Design review of the part built by this model. Coordinates are the model's own, in mm. A direction names the side the tool comes from. Round coordinates to 2 decimals unless told otherwise and drop trailing zeros. Loops run counter-clockwise (first coordinate to the right, second up) from the corner with the lowest first, then second, coordinate; pieces in that order, holes last. Notation, with made-up numbers: (81.25, 50.5) - (87.25, 50.5) arc R38 cw to (87.25, 88.5) - close; hole circle Ø5 at (70.5, -8.75). An arc over 180 degrees is marked (long way). Return JSON: item names as keys, results as strings. Group by question number.
(1) Wall thickness on L1, parallel to Y at x = -1.75, z = 18; L2, parallel to Z at x = 4.25, y = 3.25; L3, parallel to Y at x = 0.75, z = 11: over which ranges is each line inside the solid? List them lowest first. Write a range as [from, to].
(2) Clearance check with flat-ended pins moving along their axes: pin 1 (1.5 mm diameter, centred on y = -5, z = 26.5, fed in from -X); pin 2 (8 mm diameter, centred on y = 2.5, z = 21.5, fed in from +X). State where each tip first meets the part, or that it passes through.
(3) For faces 1 (the flat face through (-3.3, -5.6, 2.7)), 2 (the cylindrical face through (-0.867, -3.905, 22.558)), list the 3-axis set-ups (+Z, -Z, +X, -X, +Y, -Y) from which the entire face can be reached by the end or side of a thin tool; tool diameter is ignored.
(4) We need section A-A, the plane z = 34.5. Write out the cut boundary in (x, y), and give its area (3 significant figures).
from build123d import *

# Parameters (mm, degrees)
F1_DEPTH = 5.5
F2_R     = 4
F3_DEPTH = 35
F4_SIZE  = 0.4


with BuildPart() as f1:
    # F0 (on Top) → F1 (new body)
    with BuildSketch(Plane.XY):
        Polygon((6.5, 3.752777), (0, 7.505553), (-6.5, 3.752777), (-6.5, -3.752777), (0, -7.505553), (6.5, -3.752777), align=None)
    extrude(amount=F1_DEPTH)

    # F2 (on face) → F3 (join)
    with BuildSketch(Plane.XY.offset(5.5)):
        Circle(F2_R)
    extrude(amount=F3_DEPTH)

    # F4
    f4_edges = [f1.edges().sort_by_distance(p)[0] for p in [
        (-4, 0, 40.5),
    ]]
    chamfer(f4_edges, length=F4_SIZE)

    # F5 (on Front) → F6 (revolve, cut)
    with BuildSketch(Plane.XZ):
        Polygon((-11.5, 1), (-11.5, 0), (-6.5, 0), align=None)
    revolve(axis=Axis((0, 0, 5.5), (0, 0, -1)), mode=Mode.SUBTRACT)


solid = f1.part
Solutions:
{
 "1": {"L1": "[-3.6, 3.6]", "L2": "[0, 5.5]", "L3": "[-3.93, 3.93]"},
 "2": {"pin 1": "through", "pin 2": "x = 4"},
 "3": {"face 1": "+Z, -Z, -X, -Y", "face 2": "+Z"},
 "4": {"outline": "circle Ø8 at (0, 0)", "area": "50.3 mm^2"}
}
